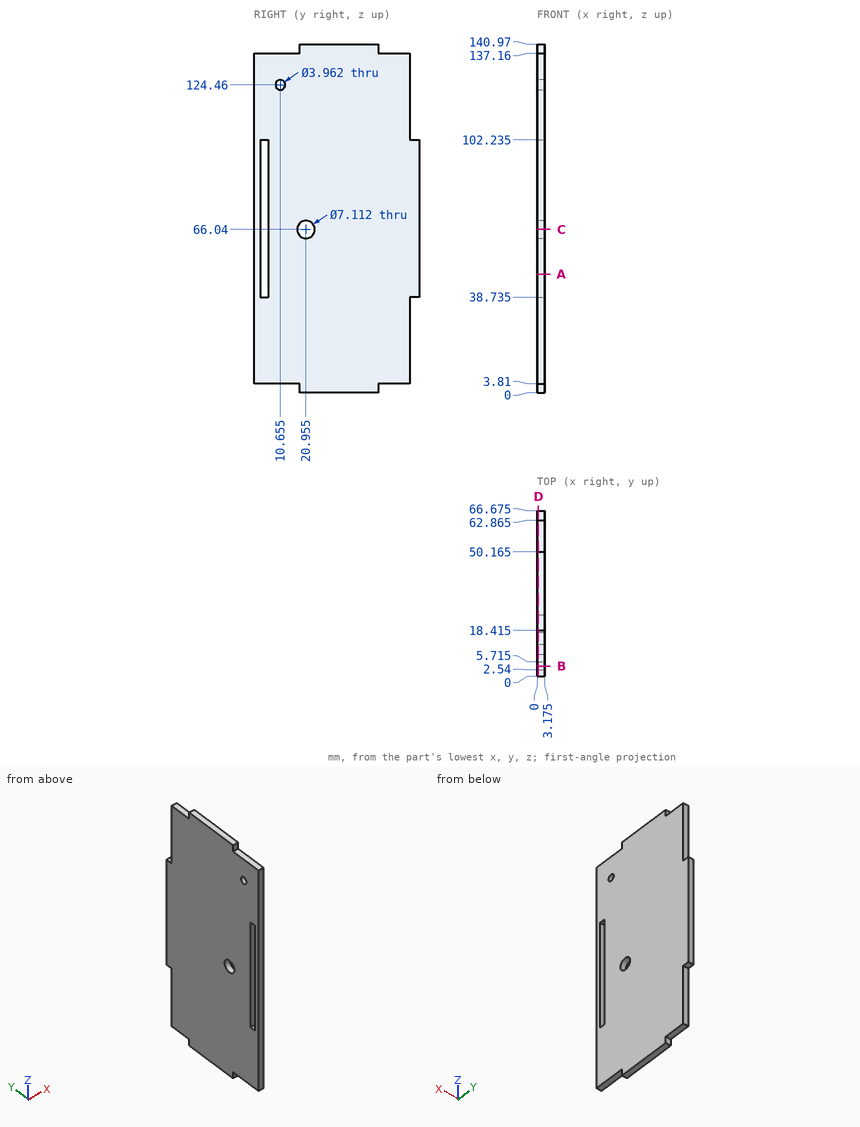
Verification items for this drawing (mm, ordinates from the low corner). Give positions to 0.01 mm unless a question says otherwise; leave off trailing zeros. Loops run counter-clockwise (first coordinate to the right, second up) from the corner with the lowest first, then second, coordinate; pieces in that order, holes last.
(1) Section check B-B on y = 4. Record the cut outline in (x, z) (1 decimal), then the cut area to 3 significant figures.
From the geometry:
outline: (0, 3.8) - (3.2, 3.8) - (3.2, 38.7) - (0, 38.7) - close; (0, 102.2) - (3.2, 102.2) - (3.2, 137.2) - (0, 137.2) - close
area: 222 mm2
(2) Section check D-D on x = 0.55. Record the cut outline in (y, z) (1 decimal).
From the geometry:
outline: (0, 3.8) - (18.4, 3.8) - (18.4, 0) - (50.2, 0) - (50.2, 3.8) - (62.9, 3.8) - (62.9, 38.7) - (66.7, 38.7) - (66.7, 102.2) - (62.9, 102.2) - (62.9, 137.2) - (50.2, 137.2) - (50.2, 141) - (18.4, 141) - (18.4, 137.2) - (0, 137.2) - close; hole (2.5, 38.7) - (5.7, 38.7) - (5.7, 102.2) - (2.5, 102.2) - close; hole circle Ø4 at (10.7, 124.5); hole circle Ø7.1 at (21, 66)
(3) Section check C-C on z = 66.04. Record the cut outline in (x, y) (1 decimal).
From the geometry:
outline: (0, 0) - (3.2, 0) - (3.2, 2.5) - (0, 2.5) - close; (0, 5.7) - (3.2, 5.7) - (3.2, 17.4) - (0, 17.4) - close; (0, 24.5) - (3.2, 24.5) - (3.2, 66.7) - (0, 66.7) - close
(4) Depth check by flat-ended pin: pin 1 Ø1.6 at (x, z) = (1.5, 22) entering from +Y (3 decimals); pin 2 Ø1.6 at (x, z) = (1.5, 2.5) entering from -Y (3 decimals); pin 3 Ø1.6 at (x, z) = (1.5, 1.5) entering from +Y (3 decimals); pin 4 Ø3 at (y, z) = (10.66, 124.46) entering from +X. Enter the tip coordinate at first touch or a pass-through.
From the geometry:
pin 1: stops at y = 62.865
pin 2: stops at y = 18.415
pin 3: stops at y = 50.165
pin 4: passes through
(5) Section check A-A on z = 48. Record the cut outline in (x, y) (1 decimal).
From the geometry:
outline: (0, 0) - (3.2, 0) - (3.2, 2.5) - (0, 2.5) - close; (0, 5.7) - (3.2, 5.7) - (3.2, 66.7) - (0, 66.7) - close
(6) Thickness scan on L1, parallel to Y at x = 1.3, z = 66.04 (1 decimal); L2, parallel to Y at x = 0.7, z = 39 (1 decimal); L3, parallel to Y at x = 1.75, z = 124.46 (1 decimal). Record the ranges inside material, lowest first.
From the geometry:
L1: y = 0 to 2.5, 5.7 to 17.4, 24.5 to 66.7
L2: y = 0 to 2.5, 5.7 to 66.7
L3: y = 0 to 8.7, 12.6 to 62.9
